```python
from build123d import *

# Parameters (mm, degrees)
BOSS_EXTRUDE1_DEPTH = 12.7
SKETCH4_R           = 2.54
CUT_EXTRUDE3_DEPTH  = 43.063657711
CUT_EXTRUDE4_DEPTH  = 43.063657711


with BuildPart() as part:
    # Sketch3 → Boss-Extrude1 (new body)
    with BuildSketch(Plane(origin=(0, 0, 0), x_dir=(1, 0, 0), z_dir=(0, 1, 0))):
        with BuildLine():
            Line((-31.75, 7.62), (6.35, 7.62))
            ThreePointArc((6.35, 7.62), (13.97, 0), (6.35, -7.62))
            Line((6.35, -7.62), (-31.75, -7.62))
            ThreePointArc((-31.75, -7.62), (-39.37, 0), (-31.75, 7.62))
        make_face()
    extrude(amount=BOSS_EXTRUDE1_DEPTH)

    # Sketch4 → Cut-Extrude3 (cut, through all)
    with BuildSketch(Plane(origin=(0, 12.7, 0), x_dir=(1, 0, 0), z_dir=(0, 1, 0))):
        with Locations(Location((-31.75, 0, 0), (0, 0, 270))):
            Circle(SKETCH4_R)
    extrude(amount=-CUT_EXTRUDE3_DEPTH, mode=Mode.SUBTRACT)

    # Sketch6 → Cut-Extrude4 (cut, through all)
    with BuildSketch(Plane(origin=(0, 12.7, 0), x_dir=(1, 0, 0), z_dir=(0, 1, 0))):
        with BuildLine():
            Line((8.00881749, 1.870380853), (4.69118251, 1.870380853))
            ThreePointArc((4.69118251, 1.870380853), (5.32458392, -2.280026724), (8.85, 0))
            ThreePointArc((8.85, 0), (8.630026724, 1.02541608), (8.00881749, 1.870380853))
        make_face()
    extrude(amount=-CUT_EXTRUDE4_DEPTH, mode=Mode.SUBTRACT)


solid = part.part
```
Model file for the job. Use its own axes, mm. A direction names the side the tool comes from. Round coordinates to 2 decimals unless told otherwise and drop trailing zeros. Loops run counter-clockwise (first coordinate to the right, second up) from the corner with the lowest first, then second, coordinate; pieces in that order, holes last. Notation, with made-up numbers: M -29,71 L 26,71 A24 cw 26,103 Z; hole C 76,45 d9. An arc over 180 degrees is marked long. Put each result on its own line as item: value. Start each with the question number.
Item 1: Cut at A-A (y = 3.5). List the corners of the cut face in (x, z).
Item 2: 3-axis set-ups, long thin cutter, end or side, ignore diameter. For faces 1 (the face through (-13, 6, -7.62)), 2 (the face through (6, 6, -1.87)): which of +Z, -Z, +X, -X, +Y, -Y reach the whole face in a straight line?
Item 3: Drop a flat-ended pin along its axis: P1, Ø2, axis at y = 6.5, z = -1.5, coming from the +X side. Give the stop position or say it passes through.
Item 4: Cut at C-C (z = -4). List the corners of the cut face in (x, y), then the cut area to 3 significant figures.
Item 5: Drill centre lines: line 1 along Z through (x, y) = (6.35, 4); line 2 along X through (y, z) = (10, 0.25); line 3 along Z through (x, y) = (7.5, 11.5). Where is each one in solid material? Low to high.
Item 6: Cut at B-B (z = 1.75). List the corners of the cut face in (x, y).
Item 7: Cut at D-D (z = 5). List the corners of the cut face in (x, y), then the cut area to 3 significant figures.
Answer block:
1. outline: M -31.75,-7.62 L 6.35,-7.62 A7.62 ccw 6.35,7.62 L -31.75,7.62 A7.62 ccw Z; hole C -31.75,0 d5.08; hole M 4.69,-1.87 L 8.01,-1.87 A2.5 ccw long Z
2. face 1: -Z, +X, -X, +Y, -Y
2. face 2: +Y, -Y
3. P1: x = 13.95
4. outline: M -38.24,0 L 12.84,0 L 12.84,12.7 L -38.24,12.7 Z
4. area: 649 mm2
5. line 1: -7.62 to -1.87, 2.5 to 7.62
5. line 2: -39.37 to -34.28, -29.22 to 3.86, 8.84 to 13.97
5. line 3: -7.53 to -1.87, 2.22 to 7.53
6. outline: M -39.17,0 L -33.59,0 L -33.59,12.7 L -39.17,12.7 Z; M -29.91,0 L 4.56,0 L 4.56,12.7 L -29.91,12.7 Z; M 8.14,0 L 13.77,0 L 13.77,12.7 L 8.14,12.7 Z
7. outline: M -37.5,0 L 12.1,0 L 12.1,12.7 L -37.5,12.7 Z
7. area: 630 mm2
